Input: part model. Units: mm. Frame: model coordinates. Face numbers are marked on the shaded views. Coordinates: 2 decimals unless noted, no trailing zeros. Order: outer loops, then holes, each group sorted by start corner. A loop starts at its lowest first (then second) coordinate and runs counter-clockwise, first axis right, second up. Notation, with made-up numbers: (17, 27.5) - (72, 27.5) arc R10 ccw to (72, 37.5) - close; hole circle Ø2 at (78.5, 34.5). An arc over 180 degrees is marked (long way). Use a Markdown table: item, result. Add a question column.
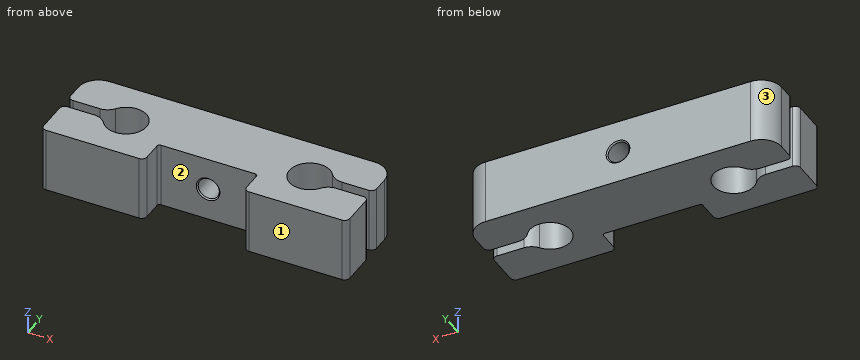
Autodesk Inventor part; units mm, degrees
ref_plane "YZ Plane" through (0, 0, 0) normal (1, 0, 0) x (0, 1, 0)
ref_plane "XZ Plane" through (0, 0, 0) normal (0, 1, 0) x (-1, 0, 0)
ref_plane "XY Plane" through (0, 0, 0) normal (0, 0, 1) x (1, 0, 0)
sketch "Sketch1" plane through (0, 0, 0) normal (0, 0, 1) x (1, 0, 0)
  line L0 (30, -9) -> (-30, -9)
  line L1 (-30, -9) -> (-30, 9)
  line L2 (-30, 9) -> (30, 9)
  line L3 (30, 9) -> (30, -9)
  line L4 (30, -9) -> (-30, 9) construction
  line L5 (-30, -9) -> (30, 9) construction
  circle A0 centre (-18, 0) radius 4
  circle A1 centre (18, 0) radius 4
  line L6 (-18, 0) -> (18, 0) construction
  line L7 (30, -1.05) -> (-30, -1.05)
  line L8 (-30, -1.05) -> (-30, 1.05) construction
  line L9 (-30, 1.05) -> (30, 1.05)
  line L10 (30, 1.05) -> (30, -1.05) construction
  line L11 (30, -1.05) -> (-30, 1.05) construction
  line L12 (-30, -1.05) -> (30, 1.05) construction
  point P0 (0, 0)
  point P1 (-21.8597, 1.05)
  point P2 (-21.8597, -1.05)
  point P3 (21.8597, -1.05)
  point P4 (21.8597, 1.05)
  dimension "d0" = 60
  dimension "d1" = 18
  dimension "d2" = 8
  dimension "d4" = 2.1
  dimension "d5" = 36
extrude "Extrusion1" add sketch "Sketch1" along normal blind 12.7 contours L0 L1 L7 A0 A1 L3 | L9 A1 A0 L1 L2 L3 | L7 A0 L9 A1
fillet "Fillet1" radius 3 4 edges at (-21.8597, 1.05, 6.35) (-21.8597, -1.05, 6.35) (21.8597, 1.05, 6.35) (21.8597, -1.05, 6.35)
sketch "Sketch2" plane through (0, 0, 12.7) normal (0, 0, 1) x (1, 0, 0)
  line L0 (9.75, -9) -> (-9.75, -9)
  line L1 (-9.75, -9) -> (-9.75, -3.725)
  line L2 (-9.75, -3.725) -> (9.75, -3.725)
  line L3 (9.75, -3.725) -> (9.75, -9)
  line L4 (9.75, -9) -> (-9.75, -3.725) construction
  line L5 (-9.75, -9) -> (9.75, -3.725) construction
  line L6 (-30, -9) -> (30, -9)
  arc A0 (-21.2625, -2.3143) -> (-21.2625, 2.3143) centre (-18, 0) ccw
  circle A1 centre (-18, 0) radius 9.052 construction
  point P0 (0, 0)
  point P1 (0, -6.3625)
  dimension "d9" = 3.725
  dimension "d10" = 5.052
  dimension "d11" = 19.5
extrude "Extrusion2" cut sketch "Sketch2" against normal up to surface (12.7 mm away)
fillet "Fillet2" radius 1 4 edges at (9.75, -9, 6.35) (-9.75, -9, 6.35) (-30, -9, 6.35) (30, -9, 6.35)
fillet "Fillet3" radius 4 2 edges at (30, 9, 6.35) (-30, 9, 6.35)
fillet "Fillet4" radius 1 4 edges at (-30, 1.05, 6.35) (-30, -1.05, 6.35) (30, 1.05, 6.35) (30, -1.05, 6.35)
fillet "Fillet5" radius 0.5 2 edges at (9.75, -3.725, 6.35) (-9.75, -3.725, 6.35)
sketch "Sketch3" plane through (-9.25, -3.725, 12.7) normal (0, -1, 0) x (1, 0, 0)
  line L0 (0, -12.7) -> (0, 0)
  line L1 (18.5, -12.7) -> (0, -12.7)
  line L2 (18.5, 0) -> (18.5, -12.7)
  line L3 (0, 0) -> (18.5, 0)
  line L4 (9.25, -12.7) -> (9.25, 0) construction
  point P0 (9.25, -6.35)
hole "Hole1" at (0, -3.725, 6.35) direction (0, 1, 0) diameter 4.134 end through all
chamfer "Chamfer1" distance 0.25 angle 45 2 edges at (0, 9, 8.417) (0, -3.725, 8.417)
properties part number "Printhead Belt Retainer" material "Aluminum 6061"
1) Cut plane C-C (y = 0). Return the cut outline in (x, z).
2) Cut plane B-B (x = 18). Return the cut outline in (y, z).
3) Material intervals for L1, parallel to Y at x = 18, z = 6.5; L2, parallel to X at y = 0, z = 6.5; L3, parallel to Y at x = 25.5, z = 7, sorted ascending.
4) Contact query for flat-ended pins moving along their axis: P1, Ø4, axis at x = -0.5, z = 3.5, coming from the -Y side (3 decimals); P2, Ø1, axis at x = -9, z = 9.5, coming from the -Y side. Output: stop coordinate, or through.
5) Cut plane A-A (y = -5). Return the cut outline in (x, z).
6) Pull-direction query (X, two-part tool) for the marked faces 1, 2 and 3; classes: pulls with the +X half, pulls with the -X half, needs draft (parallel to the pull), parting line crosses it, or undercut.
7) Cut plane D-D (x = 0). Return the cut outline in (y, z) (3 decimals), and give its area (3 significant figures).
Computed:
| question | item | result |
|---|---|---|
| 1 | outline | (-14, 0) - (14, 0) - (14, 12.7) - (-14, 12.7) - close; hole circle Ø4.13 at (0, 6.35) |
| 2 | outline | (-9, 0) - (-4, 0) - (-4, 12.7) - (-9, 12.7) - close; (4, 0) - (9, 0) - (9, 12.7) - (4, 12.7) - close |
| 3 | L1 | y = -9 to -4, 4 to 9 |
| 3 | L2 | x = -14 to -2.06, 2.06 to 14 |
| 3 | L3 | y = -9 to -1.05, 1.05 to 9 |
| 4 | P1 | stops at y = -3.725 |
| 4 | P2 | stops at y = -3.79 |
| 5 | outline | (-30, 0) - (-9.75, 0) - (-9.75, 12.7) - (-30, 12.7) - close; (9.75, 0) - (30, 0) - (30, 12.7) - (9.75, 12.7) - close |
| 6 | face 1 | needs draft |
| 6 | face 2 | undercut |
| 6 | face 3 | pulls with the -X half |
| 7 | outline | (-3.725, 0) - (9, 0) - (9, 4.033) - (8.75, 4.283) - (-3.475, 4.283) - (-3.725, 4.033) - close; (-3.725, 8.667) - (-3.475, 8.417) - (8.75, 8.417) - (9, 8.667) - (9, 12.7) - (-3.725, 12.7) - close |
| 7 | area | 109 mm2 |
